```python
from build123d import *

# Parameters (mm, degrees)
SKETCH1_W           = 50
SKETCH1_H           = 5
BOSS_EXTRUDE1_DEPTH = 50
BOSS_EXTRUDE2_DEPTH = 5
SKETCH3_R           = 5
CUT_EXTRUDE1_DEPTH  = 36


with BuildPart() as part:
    # Sketch1 → Boss-Extrude1 (new body)
    with BuildSketch(Plane.XY):
        with Locations((0, 2.5)):
            Rectangle(SKETCH1_W, SKETCH1_H)
    extrude(amount=-BOSS_EXTRUDE1_DEPTH)

    # Sketch2 → Boss-Extrude2 (add)
    with BuildSketch(Plane(origin=(5, 0, 0), x_dir=(0, 0, -1), z_dir=(1, 0, 0))):
        with BuildLine():
            Line((15, 5), (35, 5))
            Line((35, 5), (35, 13.097700543))
            ThreePointArc((35, 13.097700543), (25, 23.097700543), (15, 13.097700543))
            Line((15, 13.097700543), (15, 5))
        make_face()
    boss_extrude2 = extrude(amount=BOSS_EXTRUDE2_DEPTH)

    # Sketch3 → Cut-Extrude1 (cut, through all)
    with BuildSketch(Plane(origin=(10, 0, 0), x_dir=(0, 0, -1), z_dir=(1, 0, 0))):
        with Locations((25, 13.097700543)):
            Circle(SKETCH3_R)
    cut_extrude1 = extrude(amount=-CUT_EXTRUDE1_DEPTH, mode=Mode.SUBTRACT)

    # Mirror1: Boss-Extrude2, Cut-Extrude1 across plane
    add(boss_extrude2.mirror(Plane(origin=(0, 0, 0), x_dir=(0, 0, 1), z_dir=(1, 0, 0))))
    add(cut_extrude1.mirror(Plane(origin=(0, 0, 0), x_dir=(0, 0, 1), z_dir=(1, 0, 0))), mode=Mode.SUBTRACT)


solid = part.part
```
Build history of the part. All positions in model axes, mm. A direction names the side the tool comes from. Give positions to 0.01 mm unless a question says otherwise; leave off trailing zeros. Loops run counter-clockwise (first coordinate to the right, second up) from the corner with the lowest first, then second, coordinate; pieces in that order, holes last. Notation, with made-up numbers: (77, 86) - (110, 86) arc R17 ccw to (110, 92) - close; hole circle Ø1 at (-8.5, 30). An arc over 180 degrees is marked (long way). Use a Markdown table: item, result.
(1) Band-saw the part on B-B (y = 5.75). Give the cut face in (x, z).
Taken from the geometry:
| item | result |
|---|---|
| outline | (-10, -35) - (-5, -35) - (-5, -15) - (-10, -15) - close; (5, -35) - (10, -35) - (10, -15) - (5, -15) - close |
(2) Band-saw the part on A-A (z = -25). Give the cut face in (x, y).
Taken from the geometry:
| item | result |
|---|---|
| outline | (-25, 0) - (25, 0) - (25, 5) - (10, 5) - (10, 8.1) - (5, 8.1) - (5, 5) - (-5, 5) - (-5, 8.1) - (-10, 8.1) - (-10, 5) - (-25, 5) - close; (-10, 18.1) - (-5, 18.1) - (-5, 23.1) - (-10, 23.1) - close; (5, 18.1) - (10, 18.1) - (10, 23.1) - (5, 23.1) - close |
(3) Drop flat-ended pins along their axis: pin 1 Ø1.5 at (x, y) = (7, 11) entering from +Z; pin 2 Ø9 at (y, z) = (18, -28) entering from +X; pin 3 Ø9 at (y, z) = (10.5, -25) entering from -X. Give the stop position or say it passes through.
Taken from the geometry:
| item | result |
|---|---|
| pin 1 | z = -15 |
| pin 2 | x = 10 |
| pin 3 | x = -10 |
(4) Pull direction Z, two halves, no side cores. Call faces 4 (the face through (-7.5, 10.1, -21)), 5 (the face through (7.5, 10.1, -21)), 6 (the face through (7, 9, -35)), 7 (the face through (0, 3, 0)): +Z half, -Z half, draft (parallel to the pull), parting line (faces both ways), or undercut.
Taken from the geometry:
| item | result |
|---|---|
| face 4 | undercut |
| face 5 | undercut |
| face 6 | -Z half |
| face 7 | +Z half |
(5) Band-saw the part on C-C (x = -8.5). Give the cut face in (y, z).
Taken from the geometry:
| item | result |
|---|---|
| outline | (0, -50) - (5, -50) - (5, -35) - (13.1, -35) arc R10 ccw to (13.1, -15) - (5, -15) - (5, 0) - (0, 0) - close; hole circle Ø10 at (13.1, -25) |
(6) Which spindle directions (+Z, -Z, +X, -X, +Y, -Y) get a long thin tool onto all of the face, cutting with end or side? Do faces 1 (the face through (-7, 9, -15)), 2 (the face through (-10, 16, -20)), 3 (the face through (5, 16, -20)). Say none if no direction does.
Taken from the geometry:
| item | result |
|---|---|
| face 1 | +Z, +X, -X, +Y |
| face 2 | +Z, -Z, -X, +Y |
| face 3 | +Z, -Z, +Y |
(7) Band-saw the part on D-D (z = -17.5). Give the cut face in (x, y), and give its area (3 significant figures).
Taken from the geometry:
| item | result |
|---|---|
| outline | (-25, 0) - (25, 0) - (25, 5) - (10, 5) - (10, 19.71) - (5, 19.71) - (5, 5) - (-5, 5) - (-5, 19.71) - (-10, 19.71) - (-10, 5) - (-25, 5) - close |
| area | 397 mm2 |
(8) Wall check: line 1 along Y through (x, z) = (19.5, -17); line 2 along Y through (x, z) = (-7.75, -25); line 3 along Y through (x, z) = (7, -31). Give the ranges that are in metal, low to high.
Taken from the geometry:
| item | result |
|---|---|
| line 1 | 0 to 5 |
| line 2 | 0 to 8.1, 18.1 to 23.1 |
| line 3 | 0 to 21.1 |
